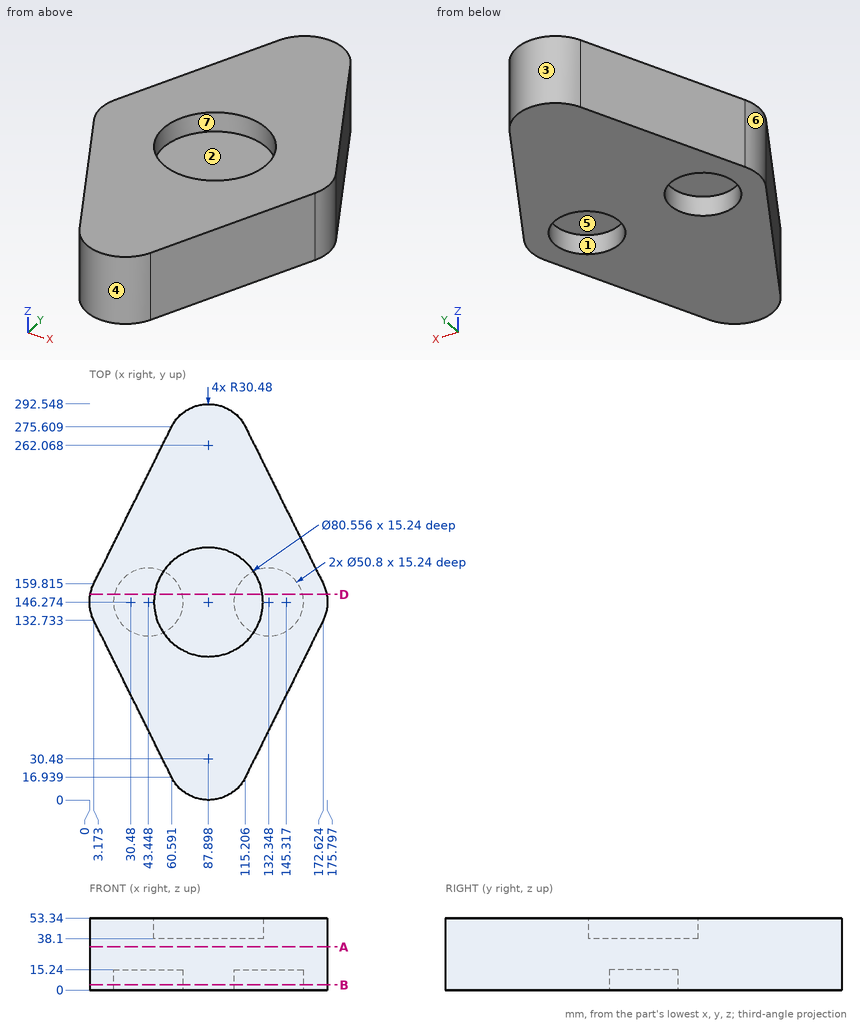
Here's the drawing with two shaded views (mm, measured from the low corner). I have some questions. A direction names the side the tool comes from. Give positions to 0.01 mm unless a question says otherwise; leave off trailing zeros. Order: outer loops, then holes, each group sorted by start corner. A loop starts at its lowest first (then second) coordinate and runs counter-clockwise, first axis right, second up. Notation, with made-up numbers: (16.25, 39) - (23.25, 39) arc R31 cw to (23.25, 68) - close; hole circle Ø8 at (57.5, -22.75). An arc over 180 degrees is marked (long way). Use a Markdown table: item, result. Add a question column.
Q1. On a 3-axis mill with a long thin cutter (end or side, diameter ignored), from which of +Z, -Z, +X, -X, +Y, -Y can I reach the whole of each face in a straight line? I mean the marked faces 5, 6 and 7. Say none if no direction works.
Q2. Please list where these lines run through material, in increasing order: line 1 along X through (y, z) = (152, 2.5) (1 decimal); line 2 along Z through (x, y) = (115, 158.5); line 3 along Y through (x, z) = (50.5, 30) (1 decimal).
Q3. If we mould it in two halves opening along Y, with no side actions, what happens to the marked faces 1, 2, 3 and 4? For each: released by +Y, released by -Y, zero draft, split by the parting line, or undercut.
Q4. If we section it at B-B on z = 4: Write out the boundary of the cut face in (x, y) (1 decimal).
Q5. I'm going to push flat-ended pins straight in: pin 1 (1.5 mm diameter, centred on x = 29.5, y = 159, fed in from -Z); pin 2 (2 mm diameter, centred on x = 153, z = 13, fed in from +Y) (1 decimal); pin 3 (3 mm diameter, centred on y = 41, z = 32.5, fed in from +X). Where does each tip first touch, or does it pass through?
Q6. If we section it at D-D on y = 152: Write out the boundary of the cut face in (x, z) (1 decimal).
Q7. If we section it at A-A on z = 32: Write out the boundary of the cut face in (x, y) (1 decimal), plus the area to 3 significant figures.
Answers follow:
| question | item | result |
|---|---|---|
| 1 | face 5 | -Z |
| 1 | face 6 | +Z, -Z, -X |
| 1 | face 7 | +Z |
| 2 | line 1 | x = 0.5 to 18.7, 68.2 to 107.6, 157.1 to 175.3 |
| 2 | line 2 | z = 15.24 to 38.1 |
| 2 | line 3 | y = 37.3 to 255.3 |
| 3 | face 1 | undercut |
| 3 | face 2 | undercut |
| 3 | face 3 | released by +Y |
| 3 | face 4 | released by -Y |
| 4 | outline | (3.2, 132.7) - (60.6, 16.9) arc R30.5 ccw to (115.2, 16.9) - (172.6, 132.7) arc R30.5 ccw to (172.6, 159.8) - (115.2, 275.6) arc R30.5 ccw to (60.6, 275.6) - (3.2, 159.8) arc R30.5 ccw to start; hole circle Ø50.8 at (43.4, 146.3); hole circle Ø50.8 at (132.3, 146.3) |
| 5 | pin 1 | stops at z = 15.24 |
| 5 | pin 2 | stops at y = 201.4 |
| 5 | pin 3 | stops at x = 127.88 |
| 6 | outline | (0.5, 0) - (18.7, 0) - (18.7, 15.2) - (68.2, 15.2) - (68.2, 0) - (107.6, 0) - (107.6, 15.2) - (157.1, 15.2) - (157.1, 0) - (175.3, 0) - (175.3, 53.3) - (127.8, 53.3) - (127.8, 38.1) - (48, 38.1) - (48, 53.3) - (0.5, 53.3) - close |
| 7 | outline | (3.2, 132.7) - (60.6, 16.9) arc R30.5 ccw to (115.2, 16.9) - (172.6, 132.7) arc R30.5 ccw to (172.6, 159.8) - (115.2, 275.6) arc R30.5 ccw to (60.6, 275.6) - (3.2, 159.8) arc R30.5 ccw to start |
| 7 | area | 32,000 mm^2 |
